```python
from build123d import *

# Parameters (mm, degrees)
SKETCH002_R  = 10
PAD001_DEPTH = 7
POCKET_DEPTH = 2
FILLET_R     = 2.5


with BuildPart() as part:
    # Sketch002 → Pad001 (new body)
    with BuildSketch(Plane.XY):
        Circle(SKETCH002_R)
    extrude(amount=PAD001_DEPTH)

    # Sketch003 → Pocket (cut)
    with BuildSketch(Plane.XY.offset(7)):
        Polygon((-1.5, 7), (1.5, 7), (1.5, 1.5), (7, 1.5), (7, -1.5), (1.5, -1.5), (1.5, -7), (-1.5, -7), (-1.5, -1.5), (-7, -1.5), (-7, 1.5), (-1.5, 1.5), align=None)
    extrude(amount=-POCKET_DEPTH, mode=Mode.SUBTRACT)

    # Fillet
    fillet_edges = [part.edges().sort_by_distance(p)[0] for p in [
        (-10, 0, 7),
    ]]
    fillet(fillet_edges, radius=FILLET_R)


solid = part.part
```
Design review of the part built by this model. Coordinates are the model's own, in mm. A direction names the side the tool comes from. Coordinates: 2 decimals unless noted, no trailing zeros. Loops run counter-clockwise (first coordinate to the right, second up) from the corner with the lowest first, then second, coordinate; pieces in that order, holes last. Notation, with made-up numbers: (30, -21) - (80, -21) arc R30 cw to (80, 12) - close; hole circle Ø8 at (-36.75, -17). An arc over 180 degrees is marked (long way). Use CSV: the item, a comma, the result in double quotes. Start each with the question number.
1) For pin 1 Ø1.6 at (y, z) = (3.5, 6.5) entering from -X; pin 2 Ø2 at (y, z) = (-2.5, 4.5) entering from +X; pin 3 Ø8 at (x, y) = (5, 5) entering from -Z; pin 4 Ø1 at (x, z) = (-0.5, 6) entering from +Y, all flat-tipped, find the tip position at first contact; note any pin that passes through.
2) Tool access review of faces 4 (the flat face through (-4, 1.5, 6)), 5 (the flat face through (0, 0, 0)): name each direction out of +Z, -Z, +X, -X, +Y, -Y from which nothing blocks a thin tool from reaching the whole face with its end or side.
3) Consider section C-C on z = 4. Write out the cut boundary in (x, y), then the cut area to 3 significant figures.
4) The part is to be moulded in two halves that separate along X. For faces 1 (the cylindrical face through (-2.17, -9.76, 2.22)), 2 (the flat face through (7, 0, 6)), 3 (the flat face through (2, -2, 7)), say which applies: +X half, -X half, draft (parallel to the pull), parting line (faces both ways), or undercut.
5) Consider section A-A on x = 0. Write out the cut boundary in (y, z), then the cut area to 3 significant figures.
6) Wall thickness on L1, parallel to X at y = 6.25, z = 6; L2, parallel to Z at x = -5.75, y = -1.25; L3, parallel to Z at x = -3.5, y = 7.75: over which ranges is each line inside the solid? List them lowest first. Write a range as from..to.
Geometry says:
1,pin 1,"x = -9.12"
1,pin 2,"x = 9.89"
1,pin 3,"z = 0"
1,pin 4,"y = 9.78"
2,face 4,"+Z"
2,face 5,"-Z, +X, -X, +Y, -Y"
3,outline,"circle Ø20 at (0, 0)"
3,area,"314 mm^2"
4,face 1,"parting line"
4,face 2,"undercut"
4,face 3,"draft"
5,outline,"(-10, 0) - (10, 0) - (10, 4.5) arc R2.5 ccw to (7.5, 7) - (7, 7) - (7, 5) - (-7, 5) - (-7, 7) - (-7.5, 7) arc R2.5 ccw to (-10, 4.5) - close"
5,area,"109 mm^2"
6,L1,"-7.15..-1.5, 1.5..7.15"
6,L2,"0..5"
6,L3,"0..6.79"
